from build123d import *

# Parameters (mm, degrees)
SKETCH_1_W          = 122.5
SKETCH_1_H          = 17
SKETCH_1_W_2        = 10
SKETCH_1_H_2        = 3
SKETCH_1_W_3        = 3
EXTRUDE_1_DEPTH     = 3
FILLET_1_R          = 1
SKETCH_2_R          = 1.5
SKETCH_2_W          = 4
SKETCH_2_H          = 1.5
SKETCH_2_W_2        = 3
SKETCH_2_H_2        = 3
CUT_EXTRUDE_1_DEPTH = 0.2


with BuildPart() as part:
    # Эскиз1 → Бобышка-Вытянуть1 (new body)
    with BuildSketch(Plane.XY):
        Rectangle(SKETCH_1_W, SKETCH_1_H)
        with Locations((0, 4)):
            Rectangle(SKETCH_1_W_2, SKETCH_1_H_2, mode=Mode.SUBTRACT)
        with Locations((57.75, -4)):
            Rectangle(SKETCH_1_W_3, SKETCH_1_H_2, mode=Mode.SUBTRACT)
        with Locations((-57.75, -4)):
            Rectangle(SKETCH_1_W_3, SKETCH_1_H_2, mode=Mode.SUBTRACT)
    extrude(amount=EXTRUDE_1_DEPTH)

    # Скругление1
    fillet_1_edges = [part.edges().sort_by_distance(p)[0] for p in [
        (61.25, -8.5, 1.5),
        (-61.25, -8.5, 1.5),
        (-61.25, 8.5, 1.5),
        (61.25, 8.5, 1.5),
    ]]
    fillet(fillet_1_edges, radius=FILLET_1_R)

    # Эскиз2 → Вырез-Вытянуть1 (cut)
    with BuildSketch(Plane.XY.offset(3)):
        with Locations((-31.944049889, 0)):
            Circle(SKETCH_2_R)
        Polygon((-22.818099779, 1.732050808), (-21.318099779, -0.866025404), (-24.318099779, -0.866025404), align=None)
        with Locations((-41.07, 0)):
            Rectangle(SKETCH_2_W, SKETCH_2_H)
        with BuildLine():
            Line((-16.192149668, -0.75), (-11.192149668, -0.75))
            ThreePointArc((-11.192149668, -0.75), (-13.692149668, 0.75), (-16.192149668, -0.75))
        make_face()
        with Locations((-4.566199557, 0)):
            Rectangle(SKETCH_2_W_2, SKETCH_2_H_2)
        Polygon((2.059750554, -1.5), (2.059750554, 1.5), (7.059750554, -1.5), align=None)
        with BuildLine():
            Line((11.953649857, -1.5), (15.417751472, -1.5))
            ThreePointArc((15.417751472, -1.5), (16.283776876, -1), (16.283776876, 0))
            ThreePointArc((16.283776876, 0), (13.685700664, 1.5), (11.087624453, 0))
            ThreePointArc((11.087624453, 0), (11.087624453, -1), (11.953649857, -1.5))
        make_face()
        with BuildLine():
            Line((21.311650775, 1), (24.311650775, 1))
            ThreePointArc((24.311650775, 1), (24.665204166, 0.853553391), (24.811650775, 0.5))
            Line((24.811650775, 0.5), (24.811650775, -0.5))
            ThreePointArc((24.811650775, -0.5), (24.665204166, -0.853553391), (24.311650775, -1))
            Line((24.311650775, -1), (21.311650775, -1))
            ThreePointArc((21.311650775, -1), (20.958097384, -0.853553391), (20.811650775, -0.5))
            Line((20.811650775, -0.5), (20.811650775, 0.5))
            ThreePointArc((20.811650775, 0.5), (20.958097384, 0.853553391), (21.311650775, 1))
        make_face()
    extrude(amount=-CUT_EXTRUDE_1_DEPTH, mode=Mode.SUBTRACT)


solid = part.part
Model file for the job. Use its own axes, mm. A direction names the side the tool comes from. Round coordinates to 2 decimals unless told otherwise and drop trailing zeros. Order: outer loops, then holes, each group sorted by start corner. A loop starts at its lowest first (then second) coordinate and runs counter-clockwise, first axis right, second up. Notation, with made-up numbers: M 67.5,-24 L 95.5,-24 A11 ccw 95.5,-8 Z; hole C -39.5,-6.75 d4. An arc over 180 degrees is marked long. Write each question's results on one line, items separated by ' | '. Start each with the question number.
(1) Two-plate mould, pull along X, no slides. Class faces 4 (the face through (59.25, -4, 1)), 5 (the face through (-58, -5.5, 1)), 6 (the face through (61.25, 0, 1)), 7 (the face through (-1, 0, 0)): pulls with the +X half, pulls with the -X half, needs draft (parallel to the pull), parting line crosses it, or undercut.
(2) Which spindle directions (+Z, -Z, +X, -X, +Y, -Y) get a long thin tool onto all of the face, cutting with end or side? Do faces 1 (the face through (-59.25, -4, 1)), 2 (the face through (-1, 0, 3)), 3 (the face through (3, -1, 2.8)). Say none if no direction does.
(3) Drop a flat-ended pin along its axis: pin 1 (0.5 mm diameter, centred on x = -14.5, y = 0, fed in from +Z). Give the stop position or say it passes through.
(4) Saw through at A-A, the plane z = 1.35. Give the cut face in (x, y), then the cut area to 3 significant figures.
(5) Probe probe 1 along Y at (x, z) = (3, 1.6); probe 2 along Y at (x, z) = (56.5, 2.25); probe 3 along X at (y, z) = (4.25, 1.3). List the from-to ranges inside material, lowest first. Write a range as from..to.
Established:
1) face 4: undercut | face 5: undercut | face 6: pulls with the +X half | face 7: needs draft
2) face 1: +Z, -Z | face 2: +Z, +X, -X, +Y, -Y | face 3: +Z
3) pin 1: stops at z = 2.8
4) outline: M -61.25,-7.5 A1 ccw -60.25,-8.5 L 60.25,-8.5 A1 ccw 61.25,-7.5 L 61.25,7.5 A1 ccw 60.25,8.5 L -60.25,8.5 A1 ccw -61.25,7.5 Z; hole M -59.25,-5.5 L -56.25,-5.5 L -56.25,-2.5 L -59.25,-2.5 Z; hole M -5,2.5 L 5,2.5 L 5,5.5 L -5,5.5 Z; hole M 56.25,-5.5 L 59.25,-5.5 L 59.25,-2.5 L 56.25,-2.5 Z | area: 2,030 mm^2
5) probe 1: y = -8.5..2.5, 5.5..8.5 | probe 2: y = -8.5..-5.5, -2.5..8.5 | probe 3: x = -61.25..-5, 5..61.25
